```python
from build123d import *

# Parameters (mm, degrees)
SKETCH1_W                        = 32.4
SKETCH1_H                        = 32.4
BOSS_EXTRUDE1_DEPTH              = 3
CBORE_FOR_M1_6_SHCS1_D           = 2.8
CBORE_FOR_M1_6_SHCS1_CBORE_D     = 5.6
CBORE_FOR_M1_6_SHCS1_CBORE_DEPTH = 1.5
SKETCH5_W                        = 18
SKETCH5_H                        = 20
CUT_EXTRUDE1_DEPTH               = 46.918623673


with BuildPart() as part:
    # Sketch1 → Boss-Extrude1 (new body)
    with BuildSketch(Plane(origin=(0, 0, 0), x_dir=(1, 0, 0), z_dir=(0, 1, 0))):
        with Locations((16.2, 16.2)):
            Rectangle(SKETCH1_W, SKETCH1_H)
    extrude(amount=BOSS_EXTRUDE1_DEPTH)

    # CBORE for M1.6 SHCS1 (through all)
    with Locations(Plane(origin=(0, 3, 0), x_dir=(1, 0, 0), z_dir=(0, 1, 0))):
        with Locations((4.2, 28.2), (28.2, 28.2), (28.2, 4.2), (4.2, 4.2)):
            CounterBoreHole(CBORE_FOR_M1_6_SHCS1_D / 2, CBORE_FOR_M1_6_SHCS1_CBORE_D / 2, CBORE_FOR_M1_6_SHCS1_CBORE_DEPTH)

    # Sketch5 → Cut-Extrude1 (cut, through all)
    with BuildSketch(Plane(origin=(0, 3, 0), x_dir=(1, 0, 0), z_dir=(0, 1, 0))):
        with Locations((16.2, 16.2)):
            Rectangle(SKETCH5_W, SKETCH5_H)
    extrude(amount=-CUT_EXTRUDE1_DEPTH, mode=Mode.SUBTRACT)


solid = part.part
```
Geometry check sheet. Reference: the model listing, model coordinates, mm. A direction names the side the tool comes from. Give positions to 0.01 mm unless a question says otherwise; leave off trailing zeros. Write each loop counter-clockwise with the first axis right and the second up, starting at its lowest first coordinate (ties: lowest second). Pieces come first, ordered by that corner, then holes.
1) Gauge pin test, flat ends, axial feed: pin 1 (8 mm diameter, centred on x = 11.5, z = -12.5, fed in from -Y); pin 2 (3 mm diameter, centred on x = 4.2, z = -4.2, fed in from +Y). Record the tip position at first contact, or that the pin passes through.
2) Section check B-B, the plane z = -28.2. Record the boundary of the cut face in (x, y).
3) Section check A-A, the plane x = 19.5. Record the boundary of the cut face in (y, z), and give its area (3 significant figures).
4) Section check D-D, the plane x = 28.2. Record the boundary of the cut face in (y, z), and give its area (3 significant figures).
5) Access from +Z, -Z, +X, -X, +Y, -Y to the whole of each face (thin tool, end or side, straight path). Record for faces 5 (the flat face through (25.2, 2, -16)), 6 (the flat face through (16, 1, -32.4)), 7 (the flat face through (29.4, 1.5, -3)).
6) Section check C-C, the plane y = 2. Record the boundary of the cut face in (x, z), and give its area (3 significant figures).
7) Material ranges on L1, parallel to Z at x = 28.2, y = 2.1; L2, parallel to Z at x = 28.2, y = 0.35; L3, parallel to X at y = 2.55, z = -28.2, recorded low to high.
8) Release check for a two-part mould opening along X. For faces 1 (the flat face through (5, 3, -16)), 2 (the flat face through (32.4, 1, -16)), 3 (the cylindrical face through (27.835, 2.26, -30.976)), 4 (the cylindrical face through (29.23, 0.74, -29.15)) record: pulls with the +X half, pulls with the -X half, needs draft (parallel to the pull), parting line crosses it, or undercut.
Computed:
1. pin 1: passes through
1. pin 2: stops at y = 1.5
2. outline: (0, 0) - (2.8, 0) - (2.8, 1.5) - (1.4, 1.5) - (1.4, 3) - (0, 3) - close; (5.6, 0) - (26.8, 0) - (26.8, 1.5) - (25.4, 1.5) - (25.4, 3) - (7, 3) - (7, 1.5) - (5.6, 1.5) - close; (29.6, 0) - (32.4, 0) - (32.4, 3) - (31, 3) - (31, 1.5) - (29.6, 1.5) - close
3. outline: (0, -32.4) - (3, -32.4) - (3, -26.2) - (0, -26.2) - close; (0, -6.2) - (3, -6.2) - (3, 0) - (0, 0) - close
3. area: 37.2 mm2
4. outline: (0, -32.4) - (3, -32.4) - (3, -31) - (1.5, -31) - (1.5, -29.6) - (0, -29.6) - close; (0, -26.8) - (1.5, -26.8) - (1.5, -25.4) - (3, -25.4) - (3, -7) - (1.5, -7) - (1.5, -5.6) - (0, -5.6) - close; (0, -2.8) - (1.5, -2.8) - (1.5, -1.4) - (3, -1.4) - (3, 0) - (0, 0) - close
4. area: 72.0 mm2
5. face 5: +Y, -Y
5. face 6: -Z, +X, -X, +Y, -Y
5. face 7: +Y
6. outline: (0, -32.4) - (32.4, -32.4) - (32.4, 0) - (0, 0) - close; hole circle Ø5.6 at (4.2, -28.2); hole circle Ø5.6 at (4.2, -4.2); hole (7.2, -26.2) - (25.2, -26.2) - (25.2, -6.2) - (7.2, -6.2) - close; hole circle Ø5.6 at (28.2, -28.2); hole circle Ø5.6 at (28.2, -4.2)
6. area: 591 mm2
7. L1: z = -32.4 to -31, -25.4 to -7, -1.4 to 0
7. L2: z = -32.4 to -29.6, -26.8 to -5.6, -2.8 to 0
7. L3: x = 0 to 1.4, 7 to 25.4, 31 to 32.4
8. face 1: needs draft
8. face 2: pulls with the +X half
8. face 3: undercut
8. face 4: undercut
